from build123d import *

# Parameters (mm, degrees)
SKETCH2_W           = 25
SKETCH2_H           = 3
BOSS_EXTRUDE1_DEPTH = 32
CIRPATTERN1_COUNT   = 6
SKETCH5_R           = 6
BOSS_EXTRUDE2_DEPTH = 32
SKETCH6_W           = 4.3
SKETCH6_H           = 4.3
AXLEHOLE_DEPTH      = 53.191951405
FILLET1_R           = 2


with BuildPart() as part:
    # Sketch1 → Revolve1 (revolve)
    with BuildSketch(Plane.XZ, mode=Mode.PRIVATE) as revolve1_sk:
        with BuildLine():
            Line((25, 0), (28, 0))
            Line((28, 0), (28, 1.5))
            Line((28, 1.5), (26.8, 1.5))
            Line((26.8, 1.5), (26.8, 4.5))
            Line((26.8, 4.5), (28, 4.5))
            Line((28, 4.5), (28, 6))
            Line((28, 6), (26.8, 6))
            Line((26.8, 6), (26.8, 28))
            Line((26.8, 28), (28, 28))
            Line((28, 28), (28, 29.5))
            Line((28, 29.5), (26.8, 29.5))
            Line((26.8, 29.5), (26.8, 32.5))
            Line((26.8, 32.5), (28, 32.5))
            Line((28, 32.5), (28, 33.999996833))
            Line((28, 33.999996833), (27, 33.999996833))
            ThreePointArc((27, 33.999996833), (25.585786438, 33.414213562), (25, 32))
            Line((25, 32), (25, 0))
        make_face()
    revolve(revolve1_sk.sketch.rotate(Axis((0, 0, 34), (0, 0, -1)), 180), axis=Axis((0, 0, 34), (0, 0, -1)))

    # Sketch2 → Boss-Extrude1 (add)
    with BuildSketch(Plane.XY):
        with Locations((12.5, 0)):
            Rectangle(SKETCH2_W, SKETCH2_H)
    boss_extrude1 = extrude(amount=BOSS_EXTRUDE1_DEPTH)

    # CirPattern1: Boss-Extrude1 ×6 about axis
    cirpattern1_axis = Axis((0, 0, 0), (0, 0, 1))
    for i in range(1, CIRPATTERN1_COUNT):
        add(boss_extrude1.rotate(cirpattern1_axis, i * 360 / CIRPATTERN1_COUNT))

    # Sketch5 → Boss-Extrude2 (add)
    with BuildSketch(Plane.XY):
        Circle(SKETCH5_R)
    extrude(amount=BOSS_EXTRUDE2_DEPTH)

    # Sketch6 → AxleHole (cut, through all)
    with BuildSketch(Plane.XY):
        Rectangle(SKETCH6_W, SKETCH6_H)
    extrude(amount=AXLEHOLE_DEPTH, mode=Mode.SUBTRACT)

    # Fillet1
    # the kernel refuses this fillet: 2 mm, written as the material it adds along each edge
    with BuildSketch(Plane(origin=(-24.954959427, -1.5, 32), x_dir=(0.10620109039764976, -0.9943446728365121, 0), z_dir=(0, 0, -1))) as fillet1_piece_1:
        with BuildLine():
            CenterArc((2.224755634, -1.997850608), FILLET1_R, 87.343441845, 98.752929077)
            Line((0.236066288, -2.210252789), (0, 0))
            ThreePointArc((0, 0), (1.158726893, 0.026867397), (2.317453785, 0))
        make_face()
    extrude(amount=32)
    with BuildSketch(Plane(origin=(-13.776517819, -20.861628814, 32), x_dir=(-0.8080272015953212, 0.589145178612228, 0), z_dir=(0, 0, -1)), Plane(origin=(13.776517819, 20.861628814, 32), x_dir=(0.8080272015953204, -0.589145178612229, 0), z_dir=(0, 0, -1)), Plane(origin=(24.954959427, -1.5, 32), x_dir=(-0.10620109039765001, -0.994344672836512, 0), z_dir=(0, 0, -1)), Plane(origin=(-11.178441608, 22.361628814, 32), x_dir=(0.9142282919929712, 0.405199494224283, 0), z_dir=(0, 0, -1)), Plane(origin=(-24.954959427, 1.5, 32), x_dir=(0.10620109039765026, 0.994344672836512, 0), z_dir=(0, 0, -1))) as fillet1_piece_2:
        with BuildLine():
            CenterArc((2.224755634, 1.997850608), FILLET1_R, 173.903629078, 98.752929077)
            Line((0.236066288, 2.210252789), (0, 0))
            ThreePointArc((0, 0), (1.158726893, -0.026867397), (2.317453785, 0))
        make_face()
    extrude(amount=32)
    with BuildSketch(Plane(origin=(-11.178441608, -22.361628814, 32), x_dir=(0.4999999999999988, 0.8660254037844393, 0), z_dir=(0, 0, -1)), Plane(origin=(13.776517819, -20.861628814, 32), x_dir=(-0.500000000000002, 0.8660254037844375, 0), z_dir=(0, 0, -1)), Plane(origin=(24.954959427, 1.5, 32), x_dir=(-1, 0, 0), z_dir=(0, 0, -1)), Plane(origin=(11.178441608, 22.361628814, 32), x_dir=(-0.5000000000000002, -0.8660254037844387, 0), z_dir=(0, 0, -1)), Plane(origin=(-13.776517819, 20.861628814, 32), x_dir=(0.5000000000000002, -0.8660254037844387, 0), z_dir=(0, 0, -1))) as fillet1_piece_3:
        with BuildLine():
            CenterArc((2.222823584, 2), FILLET1_R, 171.247070923, 98.752929077)
            ThreePointArc((0.246116119, 2.304347826), (0.096342606, 1.15502726), (0, 0))
            Line((0, 0), (2.222823584, 0))
        make_face()
    extrude(amount=32)
    with BuildSketch(Plane(origin=(5.809475019, 1.5, 32), x_dir=(1, 0, 0), z_dir=(0, 0, -1)), Plane(origin=(4.203775615, -4.281152949, 32), x_dir=(0.5000000000000001, -0.8660254037844386, 0), z_dir=(0, 0, -1)), Plane(origin=(1.605699404, 5.781152949, 32), x_dir=(0.4999999999999986, 0.8660254037844394, 0), z_dir=(0, 0, -1)), Plane(origin=(-4.203775615, 4.281152949, 32), x_dir=(-0.5000000000000004, 0.8660254037844384, 0), z_dir=(0, 0, -1)), Plane(origin=(-5.809475019, -1.5, 32), x_dir=(-1, 0, 0), z_dir=(0, 0, -1)), Plane(origin=(-1.605699404, -5.781152949, 32), x_dir=(-0.4999999999999988, -0.8660254037844393, 0), z_dir=(0, 0, -1))) as fillet1_piece_4:
        with BuildLine():
            CenterArc((1.384272266, -2), FILLET1_R, 90, 64.055520228)
            ThreePointArc((-0.414164556, -1.125), (-0.178914596, -0.572869827), (0, 0))
            Line((0, 0), (1.384272266, 0))
        make_face()
    extrude(amount=32)
    with BuildSketch(Plane(origin=(4.203775615, 4.281152949, 32), x_dir=(0.6399622417657335, -0.7684063567632539, 0), z_dir=(0, 0, -1)), Plane(origin=(5.809475019, -1.5, 32), x_dir=(-0.3454783045035584, -0.9384267372135913, 0), z_dir=(0, 0, -1)), Plane(origin=(-1.605699404, 5.781152949, 32), x_dir=(0.9854405462692932, 0.1700203804503366, 0), z_dir=(0, 0, -1)), Plane(origin=(-5.809475019, 1.5, 32), x_dir=(0.3454783045035597, 0.9384267372135907, 0), z_dir=(0, 0, -1))) as fillet1_piece_5:
        with BuildLine():
            CenterArc((1.398617439, -1.989994715), FILLET1_R, 95.733483793, 64.055520228)
            Line((-0.478236035, -1.299038106), (0, 0))
            ThreePointArc((0, 0), (0.599407474, -0.030015856), (1.198814948, 0))
        make_face()
    extrude(amount=32)
    with BuildSketch(Plane(origin=(-4.203775615, -4.281152949, 32), x_dir=(-0.4999999999999996, -0.8660254037844388, 0), z_dir=(0, 0, -1))) as fillet1_piece_6:
        with BuildLine():
            CenterArc((1.384272266, 2), FILLET1_R, 205.944479772, 64.055520228)
            ThreePointArc((-0.414164556, 1.125), (-0.178914596, 0.572869827), (0, 0))
            Line((0, 0), (1.384272266, 0))
        make_face()
    extrude(amount=32)
    # the kernel refuses this fillet: 2 mm, written as the material it takes off along each edge
    with BuildSketch(Plane(origin=(-0.894300596, -1.45102593, 32), x_dir=(0.8660254037844386, 0.5000000000000003, 0), z_dir=(0.5000000000000003, -0.8660254037844386, 0))) as fillet1_2_piece_1_section:
        with BuildLine():
            CenterArc((FILLET1_R, -FILLET1_R), FILLET1_R, 90, 90)
            Line((0, -FILLET1_R), (0, 0))
            Line((0, 0), (FILLET1_R, 0))
        make_face()
    fillet1_2_piece_1 = extrude(amount=29.145484408, mode=Mode.PRIVATE)
    fillet1_2_piece_1 = fillet1_2_piece_1 & Plane(origin=(0, 0, 32), x_dir=(-1, 0, 0), z_dir=(0, 0, -1)) * Cylinder(25, 67, mode=Mode.PRIVATE)
    fillet1_2_piece_1 = fillet1_2_piece_1 - Plane(origin=(0, 0, 32), x_dir=(1, 0, 0), z_dir=(0, 0, -1)) * Cylinder(6, 67, mode=Mode.PRIVATE)
    add(fillet1_2_piece_1, mode=Mode.SUBTRACT)


solid = part.part
Check sheet for the modelled part. Datum: model origin and axes. Units: mm. A direction names the side the tool comes from. Round coordinates to 2 decimals unless told otherwise and drop trailing zeros. One line per item, written item: value.
(1) Access from +Z, -Z, +X, -X, +Y, -Y to the whole of each face (thin tool, end or side, straight path). Record for faces 1 (the face through (5.81, -26.163, 3.021)), 2 (the face through (24.27, 2.22, 16.22)).
Computed values:
face 1: none
face 2: +Z, -Z
(2) Depth check by flat-ended pin: pin 1 Ø4 at (x, z) = (-6, 17) entering from -Y; pin 2 Ø4.5 at (x, z) = (-18.5, 14) entering from +Y; pin 3 Ø8 at (x, z) = (-12, 9) entering from -Y; pin 4 Ø8 at (x, y) = (-21.5, 0) entering from -Z. Enter the tip coordinate at first touch or a pass-through.
Computed values:
pin 1: stops at y = -26.5
pin 2: stops at y = 21.31
pin 3: stops at y = -26.39
pin 4: stops at z = 0
(3) Thickness scan on line 1 (Z direction, x = -13.5, y = -24); line 2 (X direction, y = 17.5, z = 20.5); line 3 (Y direction, x = 18.5, z = 3). Record the ranges inside material, lowest first.
Computed values:
line 1: z = 0 to 1.5, 4.5 to 6, 28 to 29.5, 32.5 to 34
line 2: x = -20.3 to -17.85, -11.84 to -8.37, 8.37 to 11.84, 17.85 to 20.3
line 3: y = -19.39 to -16.82, -1.5 to 1.5, 16.82 to 19.39
(4) Release check for a two-part mould opening along X. For faces 3 (the face through (0, -27, 29.5)), 4 (the face through (-2.15, 0, 16)), 5 (the face through (5.81, -26.163, 17.154)) record: +X half, -X half, draft (parallel to the pull), parting line (faces both ways), or undercut.
Computed values:
face 3: draft
face 4: undercut
face 5: parting line
(5) Sectioned sample at A-A, the plane y = 10. Count the separate pieces of the cut face and the enclosed holes in it, then the cut area to 3 significant figures.
Computed values:
separate pieces: 4
enclosed holes: 0
area: 368 mm^2
